```python
from build123d import *

# Parameters (mm, degrees)
SKETCH1_W           = 50.8
SKETCH1_H           = 146.685
SKETCH1_R           = 14.2494
SKETCH1_R_2         = 3.175
BOSS_EXTRUDE3_DEPTH = 6.35
SKETCH2_R           = 3.2639
CUT_EXTRUDE1_DEPTH  = 150.003260786


with BuildPart() as part:
    # Sketch1 → Boss-Extrude3 (new body)
    with BuildSketch(Plane.XY):
        with Locations((0, -73.3425)):
            Rectangle(SKETCH1_W, SKETCH1_H)
        with Locations((0, -111.76)):
            Circle(SKETCH1_R, mode=Mode.SUBTRACT)
        with Locations((-15.875, -12.7)):
            Circle(SKETCH1_R_2, mode=Mode.SUBTRACT)
        with Locations((15.875, -12.7)):
            Circle(SKETCH1_R_2, mode=Mode.SUBTRACT)
    extrude(amount=BOSS_EXTRUDE3_DEPTH)

    # Sketch2 → Cut-Extrude1 (cut, through all)
    with BuildSketch(Plane.XY.offset(6.35)):
        with Locations((8.89, -89.535)):
            Circle(SKETCH2_R)
        with Locations((-8.89, -89.535)):
            Circle(SKETCH2_R)
    extrude(amount=-CUT_EXTRUDE1_DEPTH, mode=Mode.SUBTRACT)


solid = part.part
```
Input: part model. Units: mm. Frame: model coordinates. Give positions to 0.01 mm unless a question says otherwise; leave off trailing zeros. Order: outer loops, then holes, each group sorted by start corner. A loop starts at its lowest first (then second) coordinate and runs counter-clockwise, first axis right, second up. Notation, with made-up numbers: (52.25, 71) - (58.25, 71) arc R17 ccw to (58.25, 90) - close; hole circle Ø7 at (45, -33.5). An arc over 180 degrees is marked (long way). One line per item, written item: value.
1. Cut plane D-D, the plane z = 4.25. Output: boundary loops of the cut face in (x, y) (3 decimals).
Determined:
outline: (-25.4, -146.685) - (25.4, -146.685) - (25.4, 0) - (-25.4, 0) - close; hole circle Ø6.35 at (-15.875, -12.7); hole circle Ø28.499 at (0, -111.76); hole circle Ø6.528 at (-8.89, -89.535); hole circle Ø6.528 at (8.89, -89.535); hole circle Ø6.35 at (15.875, -12.7)
2. Draft query along Y for faces 1 (the face through (0, -146.685, 3)), 2 (the face through (0, 0, 3)), 3 (the face through (10.64, -86.78, 3.22)), 4 (the face through (-25.4, -74, 3)). Return one class per face: released by +Y, released by -Y, zero draft, split by the parting line, or undercut.
Determined:
face 1: released by -Y
face 2: released by +Y
face 3: undercut
face 4: zero draft
3. Cut plane A-A, the plane y = -12.7. Output: boundary loops of the cut face in (x, z).
Determined:
outline: (-25.4, 0) - (-19.05, 0) - (-19.05, 6.35) - (-25.4, 6.35) - close; (-12.7, 0) - (12.7, 0) - (12.7, 6.35) - (-12.7, 6.35) - close; (19.05, 0) - (25.4, 0) - (25.4, 6.35) - (19.05, 6.35) - close
4. Cut plane B-B, the plane x = 0. Output: boundary loops of the cut face in (y, z) (3 decimals).
Determined:
outline: (-146.685, 0) - (-126.009, 0) - (-126.009, 6.35) - (-146.685, 6.35) - close; (-97.511, 0) - (0, 0) - (0, 6.35) - (-97.511, 6.35) - close
5. Line query: probe 1 along Y at (x, z) = (-13, 3.5) (3 decimals); probe 2 along Y at (x, z) = (10.5, 4.75) (3 decimals); probe 3 along Y at (x, z) = (0, 5) (3 decimals). Output: solid intervals per line, ascending.
Determined:
probe 1: -146.685 to -117.595, -105.925 to -14.047, -11.353 to 0
probe 2: -146.685 to -121.393, -102.127 to -92.374, -86.696 to 0
probe 3: -146.685 to -126.009, -97.511 to 0
6. Cut plane C-C, the plane y = -111.76. Output: boundary loops of the cut face in (x, z), and give its area (3 significant figures).
Determined:
outline: (-25.4, 0) - (-14.25, 0) - (-14.25, 6.35) - (-25.4, 6.35) - close; (14.25, 0) - (25.4, 0) - (25.4, 6.35) - (14.25, 6.35) - close
area: 142 mm2
